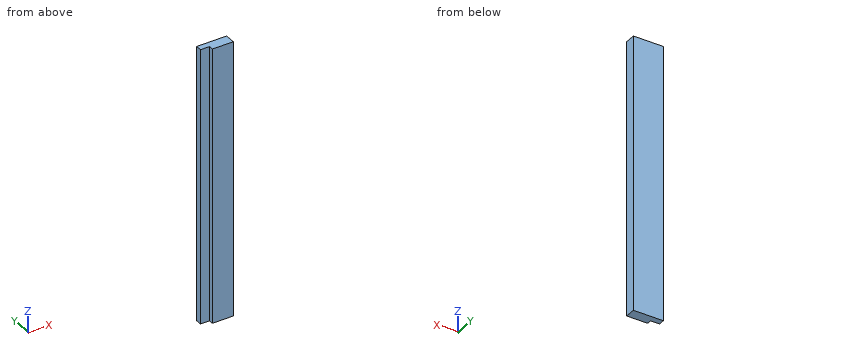
```python
from build123d import *

# Parameters (mm, degrees)
SKETCH_1_W          = 10
SKETCH_1_H          = 92
EXTRUDE_1_DEPTH     = 3.5
SKETCH_2_W          = 7
SKETCH_2_H          = 7
EXTRUDE_2_DEPTH     = 7
SKETCH_3_R          = 1.5
CUT_EXTRUDE_1_DEPTH = 7
SKETCH_4_R          = 2.15
CUT_EXTRUDE_2_DEPTH = 1
SKETCH_5_W          = 3
SKETCH_5_H          = 1.5
CUT_EXTRUDE_3_DEPTH = 92
SKETCH_6_W          = 30.020813891
SKETCH_6_H          = 96.833093315
CUT_EXTRUDE_4_DEPTH = 10


with BuildPart() as part:
    # 스케치1 → 보스-돌출1 (new body)
    with BuildSketch(Plane(origin=(0, 0, 0), x_dir=(1, 0, 0), z_dir=(0, 1, 0))):
        Rectangle(SKETCH_1_W, SKETCH_1_H)
    extrude(amount=EXTRUDE_1_DEPTH)

    # 스케치2 → 보스-돌출2 (add)
    with BuildSketch(Plane.XZ):
        with Locations((1.5, 40)):
            Rectangle(SKETCH_2_W, SKETCH_2_H)
        with Locations((1.5, 0)):
            Rectangle(SKETCH_2_W, SKETCH_2_H)
        with Locations((1.5, -40)):
            Rectangle(SKETCH_2_W, SKETCH_2_H)
    extrude(amount=EXTRUDE_2_DEPTH)

    # 스케치3 → 컷-돌출1 (cut)
    with BuildSketch(Plane(origin=(5, 0, 0), x_dir=(0, 0, -1), z_dir=(1, 0, 0))):
        with Locations((-40, -3.5)):
            Circle(SKETCH_3_R)
        with Locations((0, -3.5)):
            Circle(SKETCH_3_R)
        with Locations((40, -3.5)):
            Circle(SKETCH_3_R)
    extrude(amount=-CUT_EXTRUDE_1_DEPTH, mode=Mode.SUBTRACT)

    # 스케치4 → 컷-돌출2 (cut)
    with BuildSketch(Plane.ZY.offset(2)):
        with Locations((-40, -3.5)):
            Circle(SKETCH_4_R)
        with Locations((0, -3.5)):
            Circle(SKETCH_4_R)
        with Locations((40, -3.5)):
            Circle(SKETCH_4_R)
    extrude(amount=-CUT_EXTRUDE_2_DEPTH, mode=Mode.SUBTRACT)

    # 스케치5 → 컷-돌출3 (cut)
    with BuildSketch(Plane(origin=(0, 0, -46), x_dir=(-1, 0, 0), z_dir=(0, 0, -1))):
        with Locations((3.5, 0.75)):
            Rectangle(SKETCH_5_W, SKETCH_5_H)
    extrude(amount=-CUT_EXTRUDE_3_DEPTH, mode=Mode.SUBTRACT)

    # 스케치6 → 컷-돌출4 (cut)
    with BuildSketch(Plane.XZ):
        with Locations((-3.768545255, 0.383256933)):
            Rectangle(SKETCH_6_W, SKETCH_6_H)
    extrude(amount=CUT_EXTRUDE_4_DEPTH, mode=Mode.SUBTRACT)


solid = part.part
```
Work out the finished part from the listing and answer in its coordinate system (mm). Give positions to 0.01 mm unless a question says otherwise; leave off trailing zeros. Loops run counter-clockwise (first coordinate to the right, second up) from the corner with the lowest first, then second, coordinate; pieces in that order, holes last. Notation, with made-up numbers: (46.5, 25.25) - (95.5, 25.25) arc R24 ccw to (95.5, 49.25) - close; hole circle Ø6 at (-39.5, -9). An arc over 180 degrees is marked (long way). One line per question, with ' | ' between items.
(1) The part is cut by section C-C (y = 0.75). Write down the section's boundary in (x, z), then the cut area to 3 significant figures.
Recorded:
outline: (-2, -46) - (5, -46) - (5, 46) - (-2, 46) - close | area: 644 mm²
(2) Each of these flat-tipped pins is pushed along its axis until it touches: pin 1 Ø1.5 at (x, z) = (-1.5, 20.5) entering from -Y; pin 2 Ø2.5 at (x, z) = (-4, -10.5) entering from -Y. Where does it stop, or does it pass through?
Recorded:
pin 1: stops at y = 0 | pin 2: stops at y = 1.5
(3) Straight lines are drawn through the part: probe 1 along X at (y, z) = (0.6, 36); probe 2 along Y at (x, z) = (-4.25, -38.5). For each, find the intervals that lie inside material, in ascending order.
Recorded:
probe 1: x = -2 to 5 | probe 2: y = 1.5 to 3.5
(4) The part is cut by section B-B (x = -3.5). Write down the section's boundary in (y, z), then the cut area to 3 significant figures.
Recorded:
outline: (1.5, -46) - (3.5, -46) - (3.5, 46) - (1.5, 46) - close | area: 184 mm²
(5) The part is cut by section A-A (z = 7.5). Write down the section's boundary in (x, y).
Recorded:
outline: (-5, 1.5) - (-2, 1.5) - (-2, 0) - (5, 0) - (5, 3.5) - (-5, 3.5) - close
